Design review of the part shown in the three views and the two pictorial views. Dimensions are in mm from the part's minimum x, y and z. A direction names the side the tool comes from. Coordinates: 2 decimals unless noted, no trailing zeros. Loops run counter-clockwise (first coordinate to the right, second up) from the corner with the lowest first, then second, coordinate; pieces in that order, holes last. Notation, with made-up numbers: (-30, 10) -> (4, 10) arc R10 cw to (4, 25) -> close; hole circle Ø5 at (38.5, 77.25). An arc over 180 degrees is marked (long way). One line per item, written item: value. Start each with the question number.
1. Add section A-A on x = 5. Write out the cut boundary in (y, z).
2. Add section D-D on y = 6. Write out the cut boundary in (x, z).
3. Draft analysis for pull direction Y (two halves, no side actions). For the marked faces 4, 5 and 6, state which applies: pulls with the +Y half, pulls with the -Y half, needs draft (parallel to the pull), parting line crosses it, or undercut.
4. Add section C-C on y = 23. Write out the cut boundary in (x, z), plus the area to 3 significant figures.
5. Insertion check: pin 1 (6 mm diameter, centred on y = 22.5, z = 10, fed in from -X); pin 2 (3 mm diameter, centred on x = 30, z = 3, fed in from -Y); pin 3 (6.5 mm diameter, centred on x = 37, z = 7, fed in from +Y); pin 4 (11 mm diameter, centred on x = 21, y = 23, fed in from +Z). Each pin has a flat end and moves straight along its axis. Give the tip position at first contact, or say it passes through.
6. Machinability: for the marked faces 1, 2 and 3, which of the approach directions +Z, -Z, +X, -X, +Y, -Y give a long, thin tool a straight path to every point of the face, cutting with its end or side? Answer none if there is none.
7. Add section B-B on z = 5. Write out the cut boundary in (x, y), plus the area to 3 significant figures.
8. For probe 1 along X at (y, z) = (34, 13); probe 2 along Z at (x, y) = (37, 4); probe 3 along X at (y, z) = (23, 7.75), list the stretches that pass through material, from the lowest coordinate up.
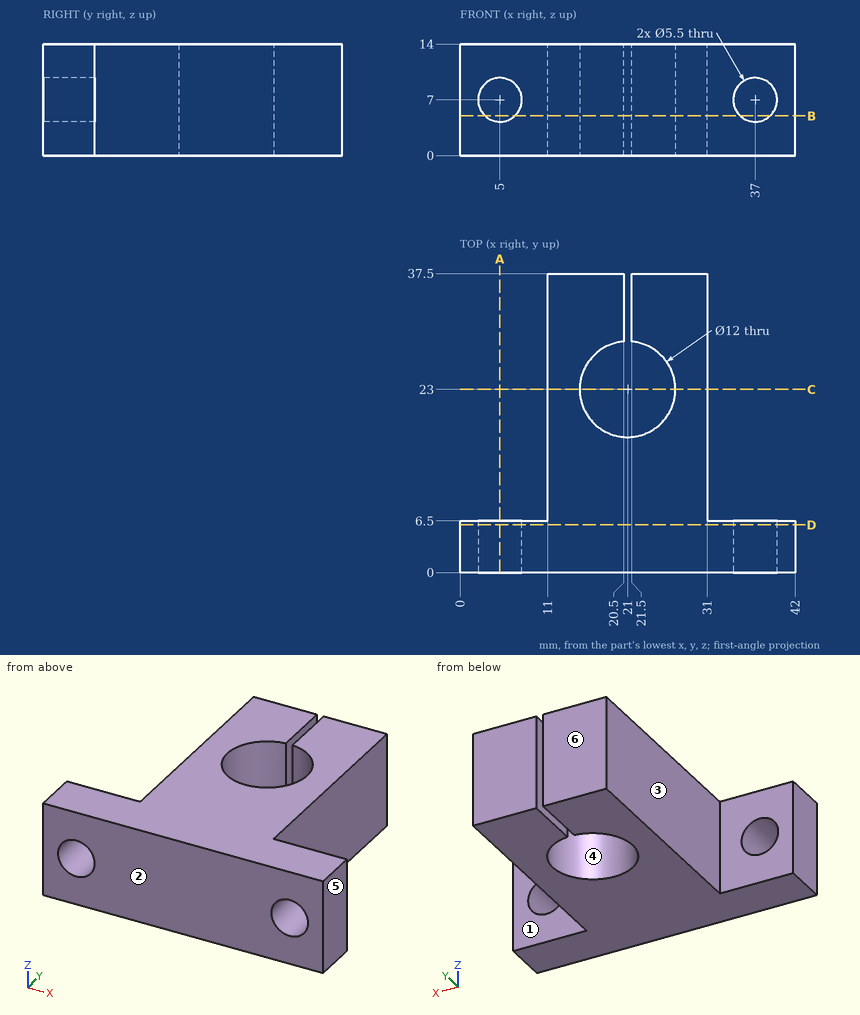
Worked answers:
1. outline: (0, 0) -> (6.5, 0) -> (6.5, 4.25) -> (0, 4.25) -> close; (0, 9.75) -> (6.5, 9.75) -> (6.5, 14) -> (0, 14) -> close
2. outline: (0, 0) -> (42, 0) -> (42, 14) -> (0, 14) -> close; hole circle Ø5.5 at (5, 7); hole circle Ø5.5 at (37, 7)
3. face 4: undercut
3. face 5: needs draft
3. face 6: pulls with the +Y half
4. outline: (11, 0) -> (15, 0) -> (15, 14) -> (11, 14) -> close; (27, 0) -> (31, 0) -> (31, 14) -> (27, 14) -> close
4. area: 112 mm²
5. pin 1: stops at x = 11
5. pin 2: stops at y = 0
5. pin 3: stops at y = 6.5
5. pin 4: passes through
6. face 1: +Z, -Z, +X, +Y
6. face 2: +Z, -Z, +X, -X, -Y
6. face 3: +Z, -Z, -X, +Y
7. outline: (0, 0) -> (3.11, 0) -> (3.11, 6.5) -> (0, 6.5) -> close; (6.89, 0) -> (35.11, 0) -> (35.11, 6.5) -> (31, 6.5) -> (31, 37.5) -> (21.5, 37.5) -> (21.5, 28.98) arc R6 cw (long way) to (20.5, 28.98) -> (20.5, 37.5) -> (11, 37.5) -> (11, 6.5) -> (6.89, 6.5) -> close; (38.89, 0) -> (42, 0) -> (42, 6.5) -> (38.89, 6.5) -> close
7. area: 722 mm²
8. probe 1: x = 11 to 20.5, 21.5 to 31
8. probe 2: z = 0 to 4.25, 9.75 to 14
8. probe 3: x = 11 to 15, 27 to 31
